Check sheet for the drawn part. Datum: minimum x, y, z corner. Units: mm. A direction names the side the tool comes from. Round coordinates to 2 decimals unless told otherwise and drop trailing zeros. Loops run counter-clockwise (first coordinate to the right, second up) from the corner with the lowest first, then second, coordinate; pieces in that order, holes last.
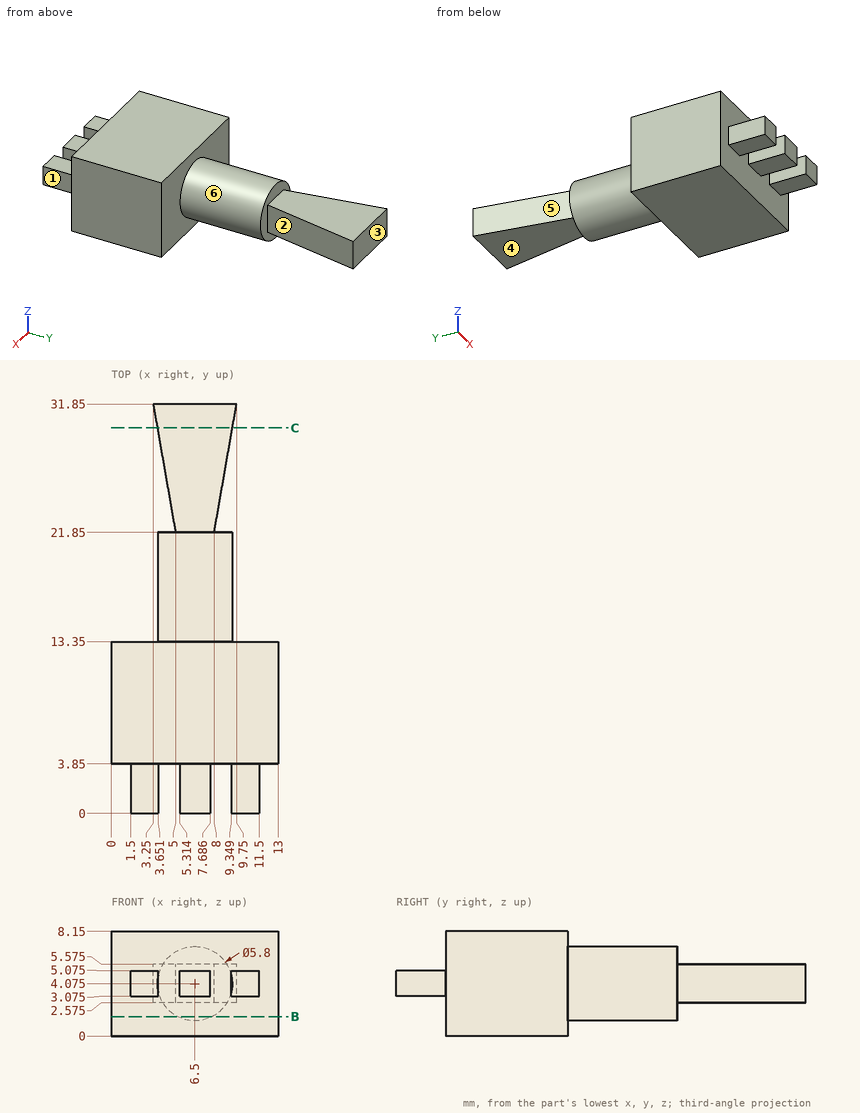
1. Scan lines: L1, parallel to X at y = 3, z = 4; L2, parallel to Y at x = 3.25, z = 2; L3, parallel to Z at x = 10.5, y = 2.5 (1 decimal). Record each from-to range of solid material in increasing order.
2. Gauge pin test, flat ends, axial feed: P1, Ø3, axis at x = 5.5, y = 26.5, coming from the +Z side (3 decimals); P2, Ø1.7, axis at x = 10.5, y = 1.5, coming from the -Z side (3 decimals); P3, Ø7, axis at x = 6, y = 28.5, coming from the -Z side (3 decimals). Record the tip position at first contact, or that the pin passes through.
3. Tool access check on the marked faces 4, 5 and 6. Record the directions out of +Z, -Z, +X, -X, +Y, -Y that give a thin tool (end or side, any length) a straight path to the whole face; none if there is none.
4. Section check C-C (y = 30). Enter the section's corners in (x, z) (1 decimal).
5. Release check for a two-part mould opening along Y. For the marked faces 1, 2 and 3 record: released by +Y, released by -Y, zero draft, split by the parting line, or undercut.
6. Section check B-B (z = 1.5). Enter the section's corners in (x, y), then the cut area to 3 significant figures.
Taken from the geometry:
1. L1: x = 1.5 to 3.65, 5.31 to 7.69, 9.35 to 11.5
1. L2: y = 3.85 to 13.35
1. L3: z = 3.1 to 5.1
2. P1: stops at z = 5.575
2. P2: stops at z = 3.075
2. P3: stops at z = 2.575
3. face 4: -Z, +X, -X, +Y
3. face 5: +Z, -Z, -X
3. face 6: none
4. outline: (3.6, 2.6) - (9.4, 2.6) - (9.4, 5.6) - (3.6, 5.6) - close
5. face 1: zero draft
5. face 2: undercut
5. face 3: released by +Y
6. outline: (0, 3.85) - (13, 3.85) - (13, 13.35) - (7.83, 13.35) - (7.83, 21.85) - (5.17, 21.85) - (5.17, 13.35) - (0, 13.35) - close
6. area: 146 mm2
